The drawing under review shows one solid part. Ordinate dimensions are in mm from its lowest x, y, z. A direction names the side the tool comes from. Coordinates: 2 decimals unless noted, no trailing zeros. Order: outer loops, then holes, each group sorted by start corner. A loop starts at its lowest first (then second) coordinate and runs counter-clockwise, first axis right, second up.
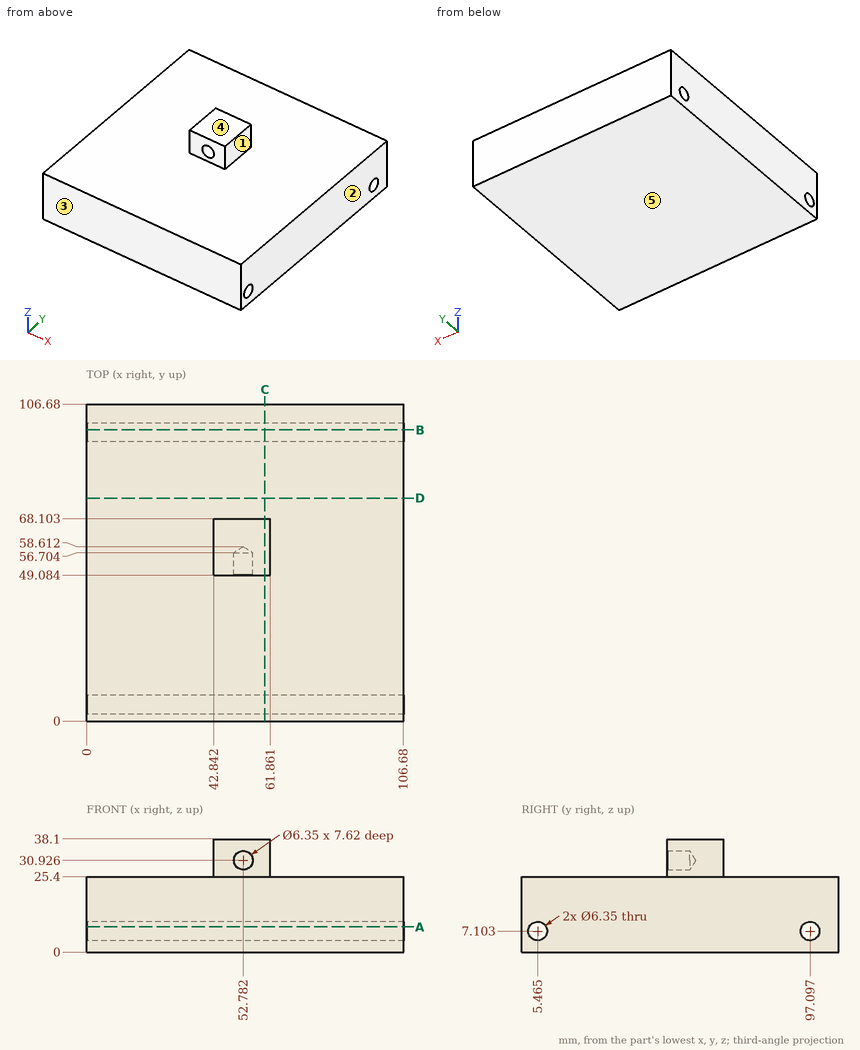
1. Clearance check with flat-ended pins moving along their axes: pin 1 Ø14 at (y, z) = (61.5, 29) entering from -X; pin 2 Ø8.5 at (x, z) = (52.78, 30.93) entering from -Y; pin 3 Ø8 at (x, y) = (92, 43) entering from +Z; pin 4 Ø10 at (x, z) = (45.5, 30.5) entering from +Y. State where each tip first meets the part, or that it passes through.
Answer below:
pin 1: stops at x = 0
pin 2: stops at y = 49.08
pin 3: stops at z = 25.4
pin 4: stops at y = 68.1
2. Machinability: for the marked faces 1 and 2, which of the approach directions +Z, -Z, +X, -X, +Y, -Y give a long, thin tool a straight path to every point of the face, cutting with its end or side? Answer none if there is none.
Answer below:
face 1: +Z, +X, +Y, -Y
face 2: +Z, -Z, +X, +Y, -Y
3. Take a section at B-B, the plane y = 98. Give the boundary of the cut face in (x, z), plus the area to 3 significant figures.
Answer below:
outline: (0, 0) - (106.68, 0) - (106.68, 4.06) - (0, 4.06) - close; (0, 10.15) - (106.68, 10.15) - (106.68, 25.4) - (0, 25.4) - close
area: 2,060 mm2
4. The part is to be moulded in two halves that separate along Z. For the marked faces 3, 4 and 5, say which applies: +Z half, -Z half, draft (parallel to the pull), parting line (faces both ways), or undercut.
Answer below:
face 3: draft
face 4: +Z half
face 5: -Z half
5. Take a section at A-A, the plane z = 8.5. Give the boundary of the cut face in (x, y) (1 decimal), plus the area to 3 significant figures.
Answer below:
outline: (0, 0) - (106.7, 0) - (106.7, 2.6) - (0, 2.6) - close; (0, 8.3) - (106.7, 8.3) - (106.7, 94.2) - (0, 94.2) - close; (0, 99.9) - (106.7, 99.9) - (106.7, 106.7) - (0, 106.7) - close
area: 10,200 mm2
6. Take a section at C-C, the plane x = 60. Give the number of separate pieces and of enclosed holes in the cut face, plus the area to 3 significant figures.
Answer below:
separate pieces: 1
enclosed holes: 2
area: 2,890 mm2
7. Take a section at D-D, the plane y = 75. Give the boundary of the cut face in (x, z).
Answer below:
outline: (0, 0) - (106.68, 0) - (106.68, 25.4) - (0, 25.4) - close
8. To check wall thickness, follow L1, parallel to Y at x = 53, z = 7.5 (1 decimal); L2, parallel to Y at x = 90, z = 7; L3, parallel to Z at x = 85.5, y = 75. State the ranges of each line that lie inside material, in increasing order.
Answer below:
L1: y = 0 to 2.3, 8.6 to 93.9, 100.2 to 106.7
L2: y = 0 to 2.29, 8.64 to 93.92, 100.27 to 106.68
L3: z = 0 to 25.4
